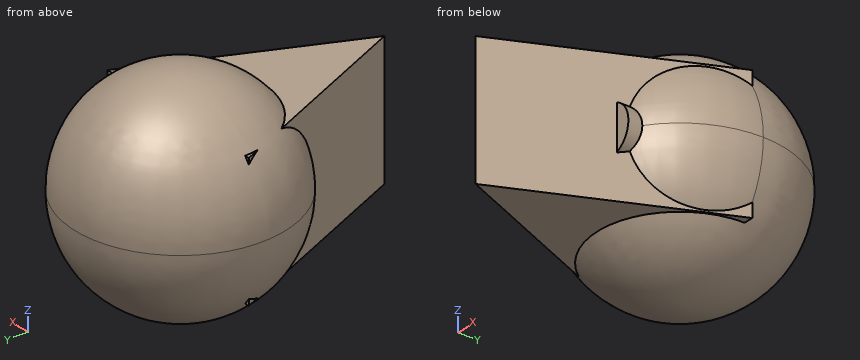
from build123d import *

# Parameters (mm, degrees)
F3_DEPTH = 8
F4_DEPTH = 8
F5_R     = 2.956664
F6_DEPTH = 12


with BuildPart() as f1:
    # F0 (on Front) → F1 (revolve)
    with BuildSketch(Plane.XZ):
        with BuildLine():
            ThreePointArc((0, -12.7), (8.980256, -8.980256), (12.7, 0))
            ThreePointArc((12.7, 0), (8.980256, 8.980256), (0, 12.7))
            Line((0, 12.7), (0, -12.7))
        make_face()
    revolve(axis=Axis((0, 0, 4.66028), (0, 0, -1)))

    # F2 (on Top) → F3 (join)
    with BuildSketch(Plane.XY):
        Polygon((11.026248, 0), (0, 0), (-10.413706, 0), (0, -24.502814), align=None)
    extrude(amount=F3_DEPTH)

    # F2 (on Top) → F4 (join)
    with BuildSketch(Plane.XY):
        Polygon((11.026248, 0), (0, 0), (-10.413706, 0), (0, -24.502814), align=None)
    extrude(amount=-F4_DEPTH)

    # F5 (on Front) → F6 (join)
    with BuildSketch(Plane.XZ):
        with Locations((4.435651, 0)):
            Circle(F5_R)
    extrude(amount=F6_DEPTH)


solid = f1.part
Geometry check sheet. Reference: the model listing, model coordinates, mm. Round coordinates to 2 decimals unless told otherwise and drop trailing zeros. Loops run counter-clockwise (first coordinate to the right, second up) from the corner with the lowest first, then second, coordinate; pieces in that order, holes last. Notation, with made-up numbers: (75.25, -30.75) -> (105.25, -30.75) arc R30 ccw to (105.25, -4.75) -> close; hole circle Ø1 at (46.5, 20). An arc over 180 degrees is marked (long way). Answer as a JSON object with one key per item and string values. Group by question number.
Item 1: Cross-section at A-A, the plane y = -17. Record the cut outline in (x, z), plus the area to 3 significant figures.
Item 2: Depth check by flat-ended pin: pin 1 Ø3 at (y, z) = (-18.5, -0.5) entering from +X; pin 2 Ø12 at (y, z) = (-3, -9) entering from +X; pin 3 Ø0.7 at (x, y) = (-10, -1) entering from -Z. Enter the tip coordinate at first touch or a pass-through.
Item 3: Thickness scan on line 1 along Y through (x, z) = (6, -8.5); line 2 along X through (y, z) = (1, -10); line 3 along Z through (x, y) = (5.5, -12). Record the ranges inside material, lowest first.
Determined:
{
 "1": {"outline": "(-3.19, -8) -> (3.38, -8) -> (3.38, 8) -> (-3.19, 8) -> close", "area": "105 mm²"},
 "2": {"pin 1": "stops at x = 3.38", "pin 2": "stops at x = 12.21", "pin 3": "stops at z = -8.2"},
 "3": {"line 1": "y = -7.28 to 7.28", "line 2": "x = -7.76 to 7.76", "line 3": "z = -8 to 8"}
}
